from build123d import *

# Parameters (mm, degrees)
ESQUISSE1_W             = 34
ESQUISSE1_H             = 24.85
BOSS_EXTRU_1_DEPTH      = 6
ESQUISSE2_R             = 1.2
ENL_V_MAT_EXTRU_1_DEPTH = 22.894762502


with BuildPart() as part:
    # Esquisse1 → Boss.-Extru.1 (new body)
    with BuildSketch(Plane.XY):
        Rectangle(ESQUISSE1_W, ESQUISSE1_H)
    extrude(amount=BOSS_EXTRU_1_DEPTH)

    # Esquisse2 → Enlèv. mat.-Extru.1 (cut, through all)
    with BuildSketch(Plane.XY.offset(6)):
        with Locations((-8, 8.005)):
            Circle(ESQUISSE2_R)
        with Locations(Location((8, 8.005, 0), (0, 0, 180))):
            Circle(ESQUISSE2_R)
        with Locations((0, 8.005)):
            Circle(ESQUISSE2_R)
        with Locations(Location((0, -8.005, 0), (0, 0, 180))):
            Circle(ESQUISSE2_R)
        with Locations((8, -8.005)):
            Circle(ESQUISSE2_R)
        with Locations(Location((-8, -8.005, 0), (0, 0, 180))):
            Circle(ESQUISSE2_R)
        with Locations((-8, 0)):
            Circle(ESQUISSE2_R)
        with Locations((8, 0)):
            Circle(ESQUISSE2_R)
    extrude(amount=-ENL_V_MAT_EXTRU_1_DEPTH, mode=Mode.SUBTRACT)


solid = part.part
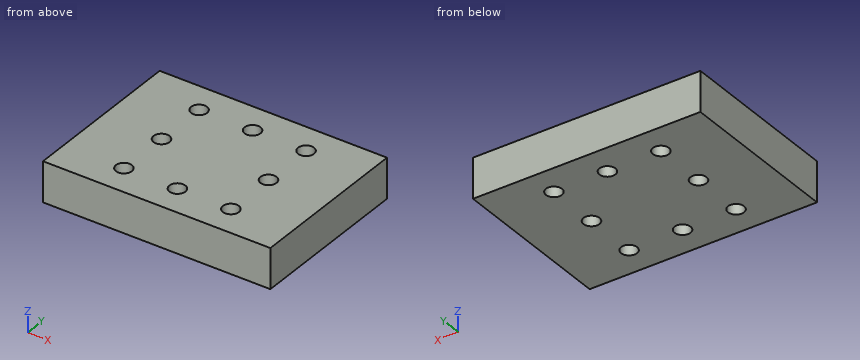
Check sheet for the modelled part. Datum: model origin and axes. Units: mm. Round coordinates to 2 decimals unless told otherwise and drop trailing zeros. Write each loop counter-clockwise with the first axis right and the second up, starting at its lowest first coordinate (ties: lowest second). Pieces come first, ordered by that corner, then holes. Notation, with made-up numbers: (86, -9.5) -> (133, -9.5) arc R14 cw to (133, 14.5) -> close; hole circle Ø8 at (-3.5, 65). An arc over 180 degrees is marked (long way). Answer as CSV lines item,"result". Start each with the question number.
1) Section check A-A on x = 0. Enter the section's corners in (y, z) (3 decimals), and give its area (3 significant figures).
2) Section check B-B on x = 8. Enter the section's corners in (y, z) (3 decimals), and give its area (3 significant figures).
3) Material ranges on line 1 (Y direction, x = 8, z = 1.35) (3 decimals); line 2 (Y direction, x = 0, z = 4.3) (3 decimals); line 3 (Y direction, x = 7.5, z = 3) (3 decimals), recorded low to high. Write a range as from..to.
4) Section check C-C on y = 0. Enter the section's corners in (x, z).
5) Go/stop test with a flat-tipped pin: P1, Ø4, axis at x = 8, y = 8.005, coming from the -Z side. Record where the tip stops, or that it passes through.
6) Section check D-D on z = 4.85. State how many separate pieces and enclosed holes the cut face has, and give its area (3 significant figures).
Found:
1,outline,"(-12.425, 0) -> (-9.205, 0) -> (-9.205, 6) -> (-12.425, 6) -> close; (-6.805, 0) -> (6.805, 0) -> (6.805, 6) -> (-6.805, 6) -> close; (9.205, 0) -> (12.425, 0) -> (12.425, 6) -> (9.205, 6) -> close"
1,area,"120 mm^2"
2,outline,"(-12.425, 0) -> (-9.205, 0) -> (-9.205, 6) -> (-12.425, 6) -> close; (-6.805, 0) -> (-1.2, 0) -> (-1.2, 6) -> (-6.805, 6) -> close; (1.2, 0) -> (6.805, 0) -> (6.805, 6) -> (1.2, 6) -> close; (9.205, 0) -> (12.425, 0) -> (12.425, 6) -> (9.205, 6) -> close"
2,area,"106 mm^2"
3,line 1,"y = -12.425..-9.205, -6.805..-1.2, 1.2..6.805, 9.205..12.425"
3,line 2,"y = -12.425..-9.205, -6.805..6.805, 9.205..12.425"
3,line 3,"y = -12.425..-9.096, -6.914..-1.091, 1.091..6.914, 9.096..12.425"
4,outline,"(-17, 0) -> (-9.2, 0) -> (-9.2, 6) -> (-17, 6) -> close; (-6.8, 0) -> (6.8, 0) -> (6.8, 6) -> (-6.8, 6) -> close; (9.2, 0) -> (17, 0) -> (17, 6) -> (9.2, 6) -> close"
5,P1,"stops at z = 0"
6,separate pieces,"1"
6,enclosed holes,"8"
6,area,"809 mm^2"
